Input: part model. Units: mm. Frame: model coordinates. A direction names the side the tool comes from. Round coordinates to 2 decimals unless told otherwise and drop trailing zeros. Order: outer loops, then holes, each group sorted by start corner. A loop starts at its lowest first (then second) coordinate and runs counter-clockwise, first axis right, second up. Notation, with made-up numbers: (13, 29) -> (38, 29) arc R31 cw to (38, 62) -> close; hole circle Ø9 at (36.5, 80.5). An arc over 180 degrees is marked (long way). Use a Markdown table: item, result.
from build123d import *

# Parameters (mm, degrees)
F0_W     = 1200
F0_H     = 1900
F0_W_2   = 350
F0_H_2   = 1675
F0_H_3   = 1673.7432479858
F1_DEPTH = 550
F2_SIZE2 = 545
F2_SIZE  = 180
F3_START = 547
F3_DEPTH = 3


with BuildPart() as f1:
    # F0 (on Front) → F1 (new body)
    with BuildSketch(Plane.XZ):
        with Locations((-575, 925)):
            Rectangle(F0_W, F0_H)
        with Locations((-975, 837.5)):
            Rectangle(F0_W_2, F0_H_2, mode=Mode.SUBTRACT)
        with Locations((-575, 837.5)):
            Rectangle(F0_W_2, F0_H_2, mode=Mode.SUBTRACT)
        with Locations((-175, 836.8716239929)):
            Rectangle(F0_W_2, F0_H_3, mode=Mode.SUBTRACT)
    extrude(amount=F1_DEPTH)

    # F2
    f2_edges = [f1.edges().sort_by_distance(p)[0] for p in [
        (-575, 0, 1875),
    ]]
    f2_side = f1.faces().sort_by_distance((-575, 0, 1852.527795))[0]
    chamfer(f2_edges, length=F2_SIZE, length2=F2_SIZE2, reference=f2_side)

    # F0 (on Front) → F3 (join)
    with BuildSketch(Plane.XZ.offset(F3_START)):
        with Locations((-575, 925)):
            Rectangle(F0_W, F0_H)
        with Locations((-975, 837.5)):
            Rectangle(F0_W_2, F0_H_2, mode=Mode.SUBTRACT)
        with Locations((-575, 837.5)):
            Rectangle(F0_W_2, F0_H_2, mode=Mode.SUBTRACT)
        with Locations((-175, 836.8716239929)):
            Rectangle(F0_W_2, F0_H_3, mode=Mode.SUBTRACT)
        with Locations((-975, 837.5)):
            Rectangle(F0_W_2, F0_H_2)
        with Locations((-575, 837.5)):
            Rectangle(F0_W_2, F0_H_2)
        with Locations((-175, 836.8716239929)):
            Rectangle(F0_W_2, F0_H_3)
    extrude(amount=F3_DEPTH)


solid = f1.part
1) Cut plane C-C on x = -999. Return loops of the section in (y, z).
Answer key:
| item | result |
|---|---|
| outline | (-550, -25) -> (0, -25) -> (0, 0) -> (-547, 0) -> (-547, 1675) -> (0, 1675) -> (0, 1695) -> (-545, 1875) -> (-550, 1875) -> close |
2) Set-up query: faces 1 (the face through (-177, -270, 1673.743)), 2 (the face through (-583, -271, -25)). Return all of +Z, -Z, +X, -X, +Y, -Y with unobstructed straight access to the full face (end or side cutting, diameter ignored); none if empty.
Answer key:
| item | result |
|---|---|
| face 1 | +Y |
| face 2 | -Z, +X, -X, +Y, -Y |
3) Cut plane A-A on z = 753. Return loops of the section in (x, y), and give its area (4 significant figures).
Answer key:
| item | result |
|---|---|
| outline | (-1175, -550) -> (25, -550) -> (25, 0) -> (0, 0) -> (0, -547) -> (-350, -547) -> (-350, 0) -> (-400, 0) -> (-400, -547) -> (-750, -547) -> (-750, 0) -> (-800, 0) -> (-800, -547) -> (-1150, -547) -> (-1150, 0) -> (-1175, 0) -> close |
| area | 85,650 mm^2 |
4) Contact query for flat-ended pins moving along their axis: P1, Ø8, axis at x = -133.5, y = -147, coming from the +Z side; P2, Ø1, axis at x = -160, y = -81.5, coming from the +Z side; P3, Ø3, axis at x = -590, z = 951, coming from the +Y side. Output: stop coordinate, or through.
Answer key:
| item | result |
|---|---|
| P1 | stops at z = 1744.87 |
| P2 | stops at z = 1722.08 |
| P3 | stops at y = -547 |
5) Cut plane B-B on y = -209.5. Return loops of the section in (x, z), and give its area (3 significant figures).
Answer key:
| item | result |
|---|---|
| outline | (-1175, -25) -> (25, -25) -> (25, 1764.19) -> (-1175, 1764.19) -> close; hole (-1150, 0) -> (-800, 0) -> (-800, 1675) -> (-1150, 1675) -> close; hole (-750, 0) -> (-400, 0) -> (-400, 1675) -> (-750, 1675) -> close; hole (-350, 0) -> (0, 0) -> (0, 1673.74) -> (-350, 1673.74) -> close |
| area | 389,000 mm^2 |
6) Draft query along X for faces 3 (the face through (-177, -270, 0)), 4 (the face through (-577, -270, 0)), 5 (the face through (25, -271, 912)), 6 (the face through (-583.4, -276.32, 1786.26)). Return one class per face: released by +X, released by -X, zero draft, split by the parting line, or undercut.
Answer key:
| item | result |
|---|---|
| face 3 | undercut |
| face 4 | undercut |
| face 5 | released by +X |
| face 6 | zero draft |
7) Cut plane D-D on y = -119. Return loops of the section in (x, z), and give its area (3 significant figures).
Answer key:
| item | result |
|---|---|
| outline | (-1175, -25) -> (25, -25) -> (25, 1734.3) -> (-1175, 1734.3) -> close; hole (-1150, 0) -> (-800, 0) -> (-800, 1675) -> (-1150, 1675) -> close; hole (-750, 0) -> (-400, 0) -> (-400, 1675) -> (-750, 1675) -> close; hole (-350, 0) -> (0, 0) -> (0, 1673.74) -> (-350, 1673.74) -> close |
| area | 353,000 mm^2 |
8) Ray query, probe 1 along X at (y, z) = (-268.5, 490); probe 2 along Y at (x, z) = (-622.5, 699); probe 3 along Z at (x, y) = (-1112, -416.5). Return the intervals inside material, ascending.
Answer key:
| item | result |
|---|---|
| probe 1 | x = -1175 to -1150, -800 to -750, -400 to -350, 0 to 25 |
| probe 2 | y = -550 to -547 |
| probe 3 | z = -25 to 0, 1675 to 1832.56 |
